Build history of the part. All positions in model axes, mm. Face numbers are marked on the shaded views. Give positions to 0.01 mm unless a question says otherwise; leave off trailing zeros. Loops run counter-clockwise (first coordinate to the right, second up) from the corner with the lowest first, then second, coordinate; pieces in that order, holes last. Notation, with made-up numbers: (39.5, 69) - (85.5, 69) arc R13 ccw to (85.5, 77) - close; hole circle Ø9 at (71.5, -7.5). An arc over 180 degrees is marked (long way). Return JSON: item names as keys, results as strings. Group by question number.
1) Slice it at A-A (z = 16). List the corners of the cut face in (x, y), and give its area (3 significant figures).
2) Slice it at B-B (x = 9). List the corners of the cut face in (y, z).
3) Drill centre lines: probe 1 along Z at (x, y) = (0, 2.35); probe 2 along Y at (x, z) = (-7, 1.5); probe 3 along X at (y, z) = (2.15, 9.5). Where is each one in solid material? Low to high. Write a range as from..to.
4) Slice it at C-C (y = 1.45). List the corners of the cut face in (x, z), and give its area (3 significant figures).
5) Slice it at D-D (x = 15). List the corners of the cut face in (y, z), and give its area (3 significant figures).
6) Drop flat-ended pins along their axis: pin 1 (1.5 mm diameter, centred on y = 1, z = -15.5, fed in from +X); pin 2 (0.5 mm diameter, centred on y = 2.5, z = 4, fed in from -X); pin 3 (0.5 mm diameter, centred on x = 0, y = 2.5, fed in from +Z). Give the stop position or say it passes through.
7) Mould opens along Z. For the marked faces 1, 2 and 3 say: released by +Z, released by -Z, zero draft, split by the parting line, or undercut.
Autodesk Inventor part; units mm, degrees
ref_plane "YZ Plane" through (0, 0, 0) normal (1, 0, 0) x (0, 1, 0)
ref_plane "XZ Plane" through (0, 0, 0) normal (0, 1, 0) x (-1, 0, 0)
ref_plane "XY Plane" through (0, 0, 0) normal (0, 0, 1) x (1, 0, 0)
sketch "Sketch1" plane through (0, 0, 0) normal (0, 1, 0) x (-1, 0, 0)
  circle A0 centre (0, 0) radius 20
  dimension "d0" = 40
extrude "Extrusion1" add sketch "Sketch1" along normal blind 2.6
sketch "Sketch2" plane through (0, 2.6, 0) normal (0, 1, 0) x (1, 0, 0)
  line L0 (10, -10) -> (-10, -10)
  line L1 (-10, -10) -> (-10, 10)
  line L2 (-10, 10) -> (10, 10)
  line L3 (10, 10) -> (10, -10)
  line L4 (10, -10) -> (-10, 10) construction
  line L5 (-10, -10) -> (10, 10) construction
  point P0 (0, 0)
  dimension "d3" = 20
  dimension "d4" = 20
extrude "Extrusion2" cut sketch "Sketch2" against normal blind 0.6
sketch "Sketch4" plane through (0, 2, 0) normal (0, 1, 0) x (1, 0, 0)
  line L0 (-6.2199, 8.694) -> (6.2369, 8.694) construction
  line L1 (6.2369, 8.694) -> (6.2369, -8.5651) construction
  line L2 (6.2369, -8.5651) -> (-6.2199, -8.5651) construction
  line L3 (-6.2199, -8.5651) -> (-6.2199, 8.694) construction
  spline S0 degree 2 poles (5.4835, -2.8345) (5.4835, -4.1124) (4.6361, -6.2782) (3.9231, -7.0047) knots 0 0 0 1 2 2 2
  spline S1 degree 2 poles (3.9231, -7.0047) (3.1832, -7.7714) (1.3268, -8.5651) (0.2103, -8.5651) knots 0 0 0 1 2 2 2
  spline S2 degree 2 poles (0.2103, -8.5651) (-0.9062, -8.5651) (-2.7492, -7.8118) (-3.4487, -7.0585) knots 0 0 0 1 2 2 2
  spline S3 degree 2 poles (-3.4487, -7.0585) (-4.3096, -6.1572) (-5.2782, -3.1304) (-5.2782, -0.9243) knots 0 0 0 1 2 2 2
  spline S4 degree 2 poles (-5.2782, -0.9243) (-5.2782, 1.2415) (-4.3904, 4.7256) (-3.4622, 6.0171) knots 0 0 0 1 2 2 2
  spline S5 degree 2 poles (-3.4622, 6.0171) (-2.5609, 7.2816) (0.291, 8.694) (2.1609, 8.694) knots 0 0 0 1 2 2 2
  spline S6 degree 2 poles (2.1609, 8.694) (2.7124, 8.694) (3.681, 8.5864) (4.0442, 8.4654) knots 0 0 0 1 2 2 2
  line L4 (4.0442, 8.4654) -> (4.0442, 6.3265)
  line L5 (4.0442, 6.3265) -> (3.95, 6.3265)
  spline S7 degree 2 poles (3.95, 6.3265) (3.6406, 6.4879) (2.5106, 6.7704) (1.8649, 6.7704) knots 0 0 0 1 2 2 2
  spline S8 degree 2 poles (1.8649, 6.7704) (-0.2067, 6.7704) (-2.7492, 3.9723) (-2.9913, 1.2281) knots 0 0 0 1 2 2 2
  spline S9 degree 2 poles (-2.9913, 1.2281) (-2.1977, 1.7796) (-0.5296, 2.385) (0.4659, 2.385) knots 0 0 0 1 2 2 2
  spline S10 degree 2 poles (0.4659, 2.385) (1.4344, 2.385) (2.8873, 1.9949) (3.681, 1.403) knots 0 0 0 1 2 2 2
  spline S11 degree 2 poles (3.681, 1.403) (4.5957, 0.7169) (5.4835, -1.4085) (5.4835, -2.8345) knots 0 0 0 1 2 2 2
  spline S12 degree 2 poles (3.2236, -2.9286) (3.2236, -1.9063) (2.6855, -0.5207) (2.0936, -0.0364) knots 0 0 0 1 2 2 2
  spline S13 degree 2 poles (2.0936, -0.0364) (1.6497, 0.3133) (0.5466, 0.542) (-0.0319, 0.542) knots 0 0 0 1 2 2 2
  spline S14 degree 2 poles (-0.0319, 0.542) (-0.8121, 0.542) (-2.2784, 0.0712) (-2.9913, -0.3727) knots 0 0 0 1 2 2 2
  spline S15 degree 2 poles (-2.9913, -0.3727) (-3.0048, -0.6149) (-3.0317, -1.0722) (-3.0317, -1.422) knots 0 0 0 1 2 2 2
  spline S16 degree 2 poles (-3.0317, -1.422) (-3.0317, -3.1439) (-2.3591, -5.2559) (-1.8479, -5.8074) knots 0 0 0 1 2 2 2
  spline S17 degree 2 poles (-1.8479, -5.8074) (-1.3771, -6.332) (-0.3547, -6.7491) (0.2237, -6.7491) knots 0 0 0 1 2 2 2
  spline S18 degree 2 poles (0.2237, -6.7491) (1.569, -6.7491) (3.2236, -4.8389) (3.2236, -2.9286) knots 0 0 0 1 2 2 2
  point P0 (0, 0)
extrude "Extrusion4" add sketch "Sketch4" along normal blind 0.6
properties part number "TopMarker1"
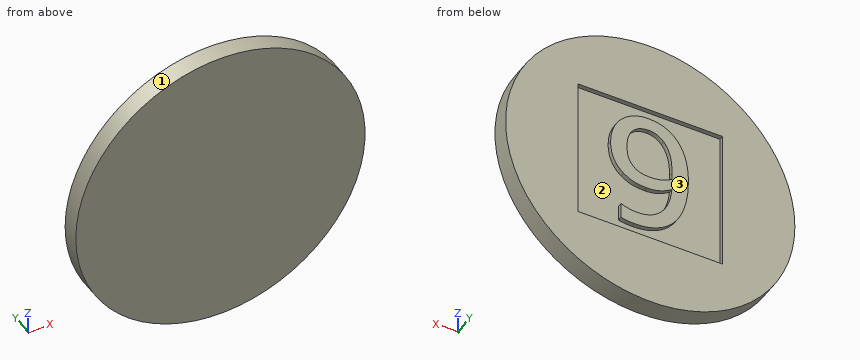
Results:
{
 "1": {"outline": "(-12, 0) - (12, 0) - (12, 2.6) - (-12, 2.6) - close", "area": "62.4 mm2"},
 "2": {"outline": "(0, -17.86) - (2.6, -17.86) - (2.6, -10) - (2, -10) - (2, 10) - (2.6, 10) - (2.6, 17.86) - (0, 17.86) - close"},
 "3": {"probe 1": "-20..-10, -8.42..-6.42, -2.37..-0.54, 6.74..8.56, 10..20", "probe 2": "0..2", "probe 3": "-17.6..-10, 10..17.6"},
 "4": {"outline": "circle Ø40 at (0, 0)", "area": "1,260 mm2"},
 "5": {"outline": "(0, -13.23) - (2.6, -13.23) - (2.6, 13.23) - (0, 13.23) - close", "area": "68.8 mm2"},
 "6": {"pin 1": "x = 13.51", "pin 2": "x = -19.65", "pin 3": "z = 20"},
 "7": {"face 1": "split by the parting line", "face 2": "undercut", "face 3": "zero draft"}
}
